Geometry: see drawing. Coordinates: mm, zero at the bounding-box minimum. Give positions to 0.01 mm unless a question says otherwise; leave off trailing zeros. Loops run counter-clockwise (first coordinate to the right, second up) from the corner with the lowest first, then second, coordinate; pieces in that order, holes last. Notation, with made-up numbers: (76.5, 57) -> (90.5, 57) arc R23 ccw to (90.5, 89) -> close; hole circle Ø10 at (6, 82.25). An arc over 180 degrees is marked (long way). Answer in a Markdown table with one row per item. Add a question column.
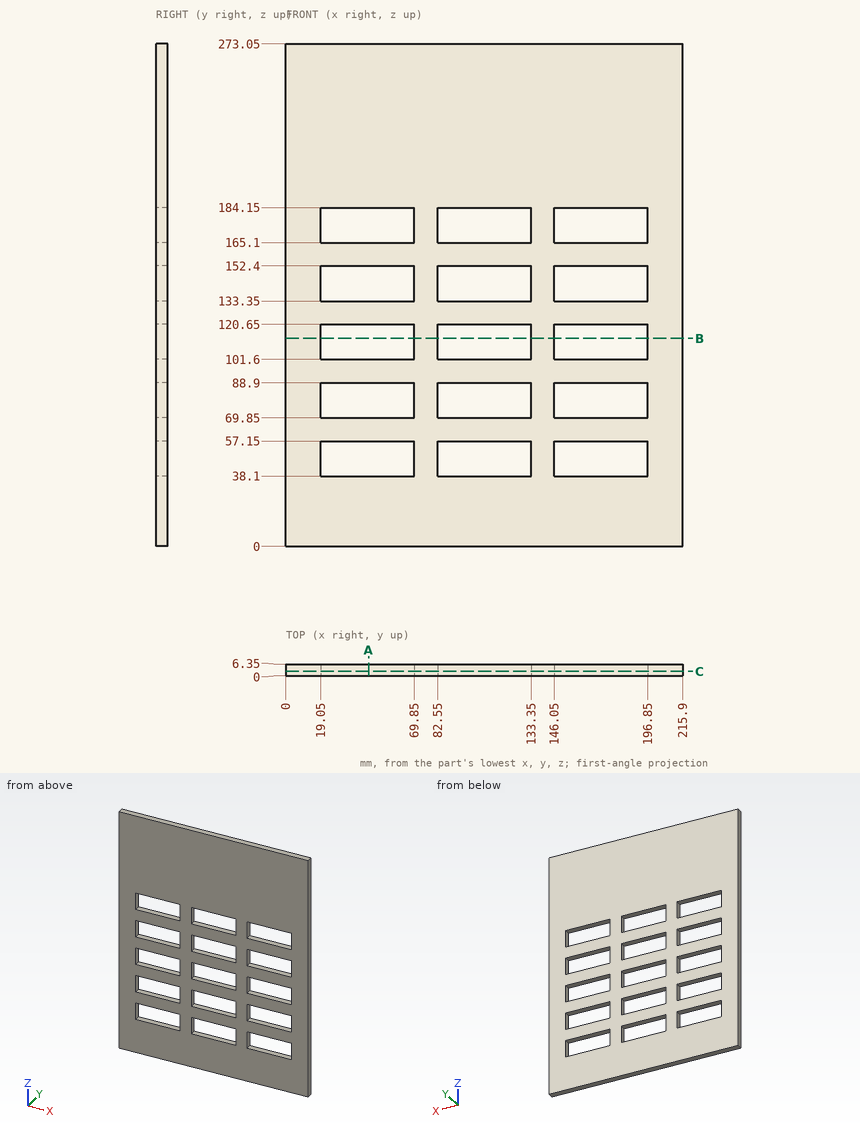
1) Section A-A on x = 45. Output: boundary loops of the cut face in (y, z).
2) Material intervals for line 1 along Z through (x, y) = (34, 0.5); line 2 along X through (y, z) = (0.75, 184), sorted ascending.
3) Section C-C on y = 2.5. State how many separate pieces and enclosed holes the cut face has, and give its area (3 significant figures).
4) Section B-B on z = 113. Output: boundary loops of the cut face in (x, y), and give its area (3 significant figures).
Working result:
| question | item | result |
|---|---|---|
| 1 | outline | (0, 0) -> (6.35, 0) -> (6.35, 38.1) -> (0, 38.1) -> close; (0, 57.15) -> (6.35, 57.15) -> (6.35, 69.85) -> (0, 69.85) -> close; (0, 88.9) -> (6.35, 88.9) -> (6.35, 101.6) -> (0, 101.6) -> close; (0, 120.65) -> (6.35, 120.65) -> (6.35, 133.35) -> (0, 133.35) -> close; (0, 152.4) -> (6.35, 152.4) -> (6.35, 165.1) -> (0, 165.1) -> close; (0, 184.15) -> (6.35, 184.15) -> (6.35, 273.05) -> (0, 273.05) -> close |
| 2 | line 1 | z = 0 to 38.1, 57.15 to 69.85, 88.9 to 101.6, 120.65 to 133.35, 152.4 to 165.1, 184.15 to 273.05 |
| 2 | line 2 | x = 0 to 19.05, 69.85 to 82.55, 133.35 to 146.05, 196.85 to 215.9 |
| 3 | separate pieces | 1 |
| 3 | enclosed holes | 15 |
| 3 | area | 44,400 mm2 |
| 4 | outline | (0, 0) -> (19.05, 0) -> (19.05, 6.35) -> (0, 6.35) -> close; (69.85, 0) -> (82.55, 0) -> (82.55, 6.35) -> (69.85, 6.35) -> close; (133.35, 0) -> (146.05, 0) -> (146.05, 6.35) -> (133.35, 6.35) -> close; (196.85, 0) -> (215.9, 0) -> (215.9, 6.35) -> (196.85, 6.35) -> close |
| 4 | area | 403 mm2 |
